Check sheet for the modelled part. Datum: model origin and axes. Units: mm. Face numbers are marked on the shaded views. A direction names the side the tool comes from. Give positions to 0.01 mm unless a question says otherwise; leave off trailing zeros. Order: outer loops, then holes, each group sorted by start corner. A loop starts at its lowest first (then second) coordinate and runs counter-clockwise, first axis right, second up. Notation, with made-up numbers: M 82.25,33.5 L 135.25,33.5 A22 ccw 135.25,58.5 Z; hole C 39.5,-4.5 d6. An arc over 180 degrees is marked long. Return JSON: item names as keys, results as strings. Group by question number.
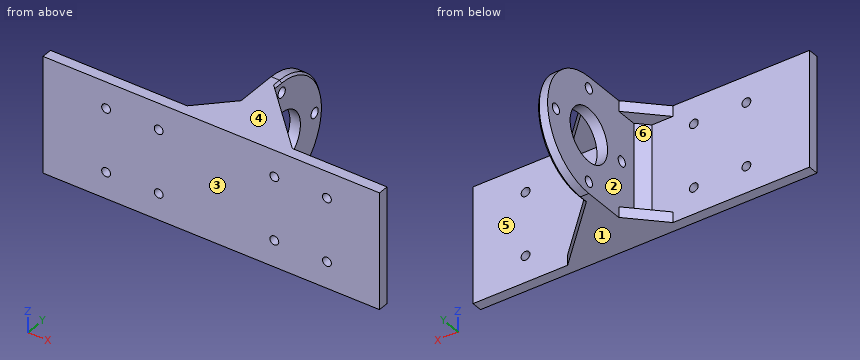
from build123d import *

# Parameters (mm, degrees)
SKETCH_1_R          = 12.5
SKETCH_1_R_2        = 2.4
EXTRUDE_1_DEPTH     = 5
SKETCH_2_W          = 55
SKETCH_2_H          = 5
EXTRUDE_2_DEPTH     = 80
RIB_1_REACH         = 105.712
SKETCH_3_WALL_W     = 230.637888562
SKETCH_3_WALL_H     = 5
CHAMFER_2_SIZE      = 5
SKETCH_4_W          = 55
SKETCH_4_H          = 5
EXTRUDE_3_DEPTH     = 75
RIB_6_REACH         = 105.712
SKETCH_5_WALL_W     = 251.851091998
SKETCH_5_WALL_H     = 5
CUT_EXTRUDE_1_REACH = 107.178
SKETCH_6_R          = 2.1
CHAMFER_3_SIZE      = 1


with BuildPart() as part:
    # 草图1 → 凸台-拉伸1 (new body)
    with BuildSketch(Plane(origin=(0, 0, 0), x_dir=(0, 0, -1), z_dir=(1, 0, 0))):
        with BuildLine():
            Line((-27.5, 0), (-27.5, -40))
            Line((-27.5, -40), (27.5, -40))
            Line((27.5, -40), (27.5, 0))
            ThreePointArc((27.5, 0), (0, 27.5), (-27.5, 0))
        make_face()
        Circle(SKETCH_1_R, mode=Mode.SUBTRACT)
        with Locations((0, 22)):
            Circle(SKETCH_1_R_2, mode=Mode.SUBTRACT)
        with Locations((22, 0)):
            Circle(SKETCH_1_R_2, mode=Mode.SUBTRACT)
        with Locations((0, -22)):
            Circle(SKETCH_1_R_2, mode=Mode.SUBTRACT)
        with Locations((-22, 0)):
            Circle(SKETCH_1_R_2, mode=Mode.SUBTRACT)
    extrude(amount=EXTRUDE_1_DEPTH)

    # 草图2 → 凸台-拉伸2 (add)
    with BuildSketch(Plane.ZY):
        with Locations((0, -37.5)):
            Rectangle(SKETCH_2_W, SKETCH_2_H)
    extrude(amount=EXTRUDE_2_DEPTH)

    # 草图3 wall → 筋1 (add, up to next)
    with BuildSketch(Plane(origin=(-7.5, -27.5, 25), x_dir=(0.707106781187, 0.707106781187, 0), z_dir=(-0.707106781187, 0.707106781187, 0)), mode=Mode.PRIVATE) as rib_1_sk1:
        Rectangle(SKETCH_3_WALL_W, SKETCH_3_WALL_H)
    rib_1_tool1 = extrude(rib_1_sk1.sketch, amount=-RIB_1_REACH, mode=Mode.PRIVATE) - part.part
    rib_1 = rib_1_tool1.solids().sort_by_distance((-7.5, -27.5, 25))[0]
    add(rib_1)

    # 镜向1: 筋1 across plane
    add(rib_1.mirror(Plane.XY))

    # 倒角2
    chamfer_2_edges = [part.edges().sort_by_distance(p)[0] for p in [
        (0, -35, 0),
    ]]
    chamfer(chamfer_2_edges, length=CHAMFER_2_SIZE)

    # 草图4 → 凸台-拉伸3 (add)
    with BuildSketch(Plane(origin=(5, 0, 0), x_dir=(0, 0, -1), z_dir=(1, 0, 0))):
        with Locations((0, -37.5)):
            Rectangle(SKETCH_4_W, SKETCH_4_H)
    extrude(amount=EXTRUDE_3_DEPTH)

    # 草图5 wall → 筋6 (add, up to next)
    with BuildSketch(Plane(origin=(20, -20, 25), x_dir=(-0.707106781187, 0.707106781187, 0), z_dir=(-0.707106781187, -0.707106781187, 0)), mode=Mode.PRIVATE) as rib_6_sk1:
        Rectangle(SKETCH_5_WALL_W, SKETCH_5_WALL_H)
    rib_6_tool1 = extrude(rib_6_sk1.sketch, amount=RIB_6_REACH, mode=Mode.PRIVATE) - part.part
    rib_6 = rib_6_tool1.solids().sort_by_distance((20, -20, 25))[0]
    add(rib_6)

    # 镜向2: 筋6 across plane
    add(rib_6.mirror(Plane.XY))

    # 草图6 → 切除-拉伸1 (cut, up to next)
    with BuildSketch(Plane(origin=(0, -35, 0), x_dir=(1, 0, 0), z_dir=(0, 1, 0)), mode=Mode.PRIVATE) as cut_extrude_1_sk1:
        with Locations(Location((30, 15, 0), (0, 0, 270))):
            Circle(SKETCH_6_R)
    cut_extrude_1_tool1 = extrude(cut_extrude_1_sk1.sketch, amount=-CUT_EXTRUDE_1_REACH, mode=Mode.PRIVATE) & part.part
    # 草图6 → 切除-拉伸1 (cut, up to next)
    with BuildSketch(Plane(origin=(0, -35, 0), x_dir=(1, 0, 0), z_dir=(0, 1, 0)), mode=Mode.PRIVATE) as cut_extrude_1_sk2:
        with Locations(Location((55, 15, 0), (0, 0, 270))):
            Circle(SKETCH_6_R)
    cut_extrude_1_tool2 = extrude(cut_extrude_1_sk2.sketch, amount=-CUT_EXTRUDE_1_REACH, mode=Mode.PRIVATE) & part.part
    # 草图6 → 切除-拉伸1 (cut, up to next)
    with BuildSketch(Plane(origin=(0, -35, 0), x_dir=(1, 0, 0), z_dir=(0, 1, 0)), mode=Mode.PRIVATE) as cut_extrude_1_sk3:
        with Locations(Location((-50, 15, 0), (0, 0, 270))):
            Circle(SKETCH_6_R)
    cut_extrude_1_tool3 = extrude(cut_extrude_1_sk3.sketch, amount=-CUT_EXTRUDE_1_REACH, mode=Mode.PRIVATE) & part.part
    # 草图6 → 切除-拉伸1 (cut, up to next)
    with BuildSketch(Plane(origin=(0, -35, 0), x_dir=(1, 0, 0), z_dir=(0, 1, 0)), mode=Mode.PRIVATE) as cut_extrude_1_sk4:
        with Locations(Location((-25, 15, 0), (0, 0, 270))):
            Circle(SKETCH_6_R)
    cut_extrude_1_tool4 = extrude(cut_extrude_1_sk4.sketch, amount=-CUT_EXTRUDE_1_REACH, mode=Mode.PRIVATE) & part.part
    # 草图6 → 切除-拉伸1 (cut, up to next)
    with BuildSketch(Plane(origin=(0, -35, 0), x_dir=(1, 0, 0), z_dir=(0, 1, 0)), mode=Mode.PRIVATE) as cut_extrude_1_sk5:
        with Locations(Location((55, -15, 0), (0, 0, 270))):
            Circle(SKETCH_6_R)
    cut_extrude_1_tool5 = extrude(cut_extrude_1_sk5.sketch, amount=-CUT_EXTRUDE_1_REACH, mode=Mode.PRIVATE) & part.part
    # 草图6 → 切除-拉伸1 (cut, up to next)
    with BuildSketch(Plane(origin=(0, -35, 0), x_dir=(1, 0, 0), z_dir=(0, 1, 0)), mode=Mode.PRIVATE) as cut_extrude_1_sk6:
        with Locations(Location((30, -15, 0), (0, 0, 270))):
            Circle(SKETCH_6_R)
    cut_extrude_1_tool6 = extrude(cut_extrude_1_sk6.sketch, amount=-CUT_EXTRUDE_1_REACH, mode=Mode.PRIVATE) & part.part
    # 草图6 → 切除-拉伸1 (cut, up to next)
    with BuildSketch(Plane(origin=(0, -35, 0), x_dir=(1, 0, 0), z_dir=(0, 1, 0)), mode=Mode.PRIVATE) as cut_extrude_1_sk7:
        with Locations(Location((-25, -15, 0), (0, 0, 270))):
            Circle(SKETCH_6_R)
    cut_extrude_1_tool7 = extrude(cut_extrude_1_sk7.sketch, amount=-CUT_EXTRUDE_1_REACH, mode=Mode.PRIVATE) & part.part
    # 草图6 → 切除-拉伸1 (cut, up to next)
    with BuildSketch(Plane(origin=(0, -35, 0), x_dir=(1, 0, 0), z_dir=(0, 1, 0)), mode=Mode.PRIVATE) as cut_extrude_1_sk8:
        with Locations(Location((-50, -15, 0), (0, 0, 270))):
            Circle(SKETCH_6_R)
    cut_extrude_1_tool8 = extrude(cut_extrude_1_sk8.sketch, amount=-CUT_EXTRUDE_1_REACH, mode=Mode.PRIVATE) & part.part
    add(cut_extrude_1_tool1.solids().sort_by_distance((30, -35, -15))[0], mode=Mode.SUBTRACT)
    add(cut_extrude_1_tool2.solids().sort_by_distance((55, -35, -15))[0], mode=Mode.SUBTRACT)
    add(cut_extrude_1_tool3.solids().sort_by_distance((-50, -35, -15))[0], mode=Mode.SUBTRACT)
    add(cut_extrude_1_tool4.solids().sort_by_distance((-25, -35, -15))[0], mode=Mode.SUBTRACT)
    add(cut_extrude_1_tool5.solids().sort_by_distance((55, -35, 15))[0], mode=Mode.SUBTRACT)
    add(cut_extrude_1_tool6.solids().sort_by_distance((30, -35, 15))[0], mode=Mode.SUBTRACT)
    add(cut_extrude_1_tool7.solids().sort_by_distance((-25, -35, 15))[0], mode=Mode.SUBTRACT)
    add(cut_extrude_1_tool8.solids().sort_by_distance((-50, -35, 15))[0], mode=Mode.SUBTRACT)

    # 倒角3
    chamfer_3_edges = [part.edges().sort_by_distance(p)[0] for p in [
        (5, -2.5, -27.5),
        (5, 27.5, 0),
        (5, -2.5, 27.5),
    ]]
    chamfer(chamfer_3_edges, length=CHAMFER_3_SIZE)


solid = part.part
1) Sectioned sample at D-D on z = -15. State how many separate pieces and enclosed holes the cut face has, then the cut area to 3 significant figures.
2) Material ranges on line 1 along X through (y, z) = (-36.2, -15); line 2 along Y through (x, z) = (-32, -13); line 3 along X through (y, z) = (16, 7.5), recorded low to high.
3) Tool access check on the marked faces 4, 5 and 6. Record the directions out of +Z, -Z, +X, -X, +Y, -Y that give a thin tool (end or side, any length) a straight path to the whole face; none if there is none.
4) Sectioned sample at B-B on y = -22. Record the boundary of the cut face in (x, z), then the cut area to 3 significant figures.
5) Depth check by flat-ended pin: P1, Ø5.5, axis at y = 0, z = -22, coming from the +X side; P2, Ø10, axis at y = -30.5, z = -14.5, coming from the +X side; P3, Ø6.5, axis at x = -25, z = -15, coming from the +Y side. Enter the tip coordinate at first touch or a pass-through.
6) Release check for a two-part mould opening along Z. For the marked faces 1, 2 and 3 record: released by +Z, released by -Z, zero draft, split by the parting line, or undercut.
7) Sectioned sample at A-A on x = 30. Record the boundary of the cut face in (y, z).
8) Sectioned sample at C-C on x = 10. Record the boundary of the cut face in (y, z), then the cut area to 3 significant figures.
Reply:
{
 "1": {"separate pieces": "5", "enclosed holes": "0", "area": "1,020 mm^2"},
 "2": {"line 1": "-80 to -52.1, -47.9 to -27.1, -22.9 to 27.9, 32.1 to 52.9, 57.1 to 80", "line 2": "-40 to -35", "line 3": "0 to 5"},
 "3": {"face 4": "+Z, +X, -X, +Y, -Y", "face 5": "+X, +Y", "face 6": "-X, +Y"},
 "4": {"outline": "M -2,-27.5 L 22,-27.5 L 22,-22.5 L 5,-22.5 L 5,-2.4 L 0,-2.4 L 0,-22.5 L -2,-22.5 Z; M -2,22.5 L 0,22.5 L 0,2.4 L 5,2.4 L 5,22.5 L 22,22.5 L 22,27.5 L -2,27.5 Z", "area": "441 mm^2"},
 "5": {"P1": "x = 5", "P2": "x = 80", "P3": "y = -35"},
 "6": {"face 1": "released by -Z", "face 2": "undercut", "face 3": "zero draft"},
 "7": {"outline": "M -40,-27.5 L -30,-27.5 L -30,-22.5 L -35,-22.5 L -35,-17.1 L -40,-17.1 Z; M -40,-12.9 L -35,-12.9 L -35,12.9 L -40,12.9 Z; M -40,17.1 L -35,17.1 L -35,22.5 L -30,22.5 L -30,27.5 L -40,27.5 Z"},
 "8": {"outline": "M -40,-27.5 L -10,-27.5 L -10,-22.5 L -35,-22.5 L -35,22.5 L -10,22.5 L -10,27.5 L -40,27.5 Z", "area": "525 mm^2"}
}
